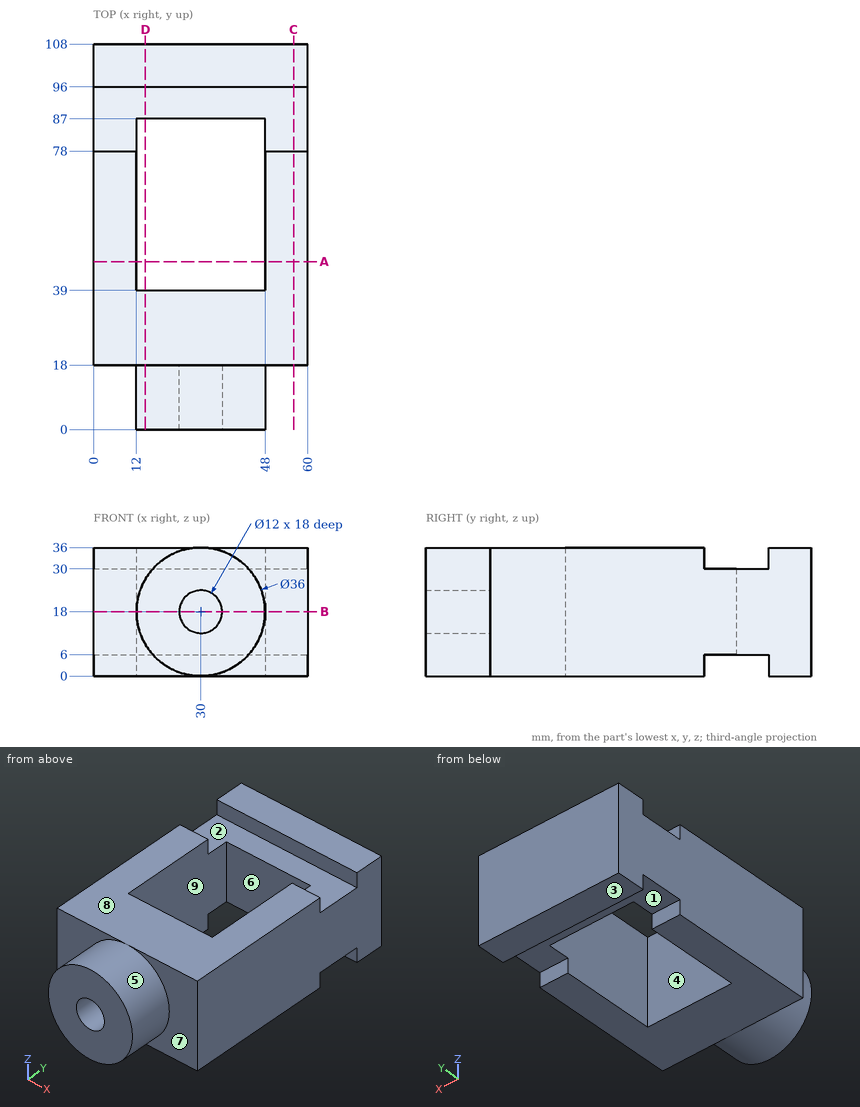
For this review, use the dimensioned drawing (mm, ordinates from the lowest corner) and the shaded views. A direction names the side the tool comes from. Coordinates: 2 decimals unless noted, no trailing zeros. Write each loop counter-clockwise with the first axis right and the second up, starting at its lowest first coordinate (ties: lowest second). Pieces come first, ordered by that corner, then holes. Notation, with made-up numbers: (-36.75, 25) - (16.25, 25) arc R26 cw to (16.25, 62) - close; hole circle Ø4 at (58.5, 24). An arc over 180 degrees is marked (long way). One line per item, written item: value.
1) Add section D-D (x = 14.5). State the section outline as (y, z) points, plus the area to 3 significant figures.
Answer sheet:
outline: (0, 8.85) - (18, 8.85) - (18, 0) - (39, 0) - (39, 36) - (18, 36) - (18, 27.15) - (0, 27.15) - close; (87, 6) - (96, 6) - (96, 0) - (108, 0) - (108, 36) - (96, 36) - (96, 30) - (87, 30) - close
area: 1,730 mm2
2) For the marked faces 1, 2, 3, 4 and 5, list the 3-axis set-ups (+Z, -Z, +X, -X, +Y, -Y) from which the entire face can be reached by the end or side of a thin tool; tool diameter is ignored.
Answer sheet:
face 1: -Z, +X, -X
face 2: +Z, +X, -X
face 3: -Z, +X, -X, +Y, -Y
face 4: +Z, -Z
face 5: -Y
3) Add section C-C (x = 56). State the section outline as (y, z) points, plus the area to 3 significant figures.
Answer sheet:
outline: (18, 0) - (78, 0) - (78, 6) - (96, 6) - (96, 0) - (108, 0) - (108, 36) - (96, 36) - (96, 30) - (78, 30) - (78, 36) - (18, 36) - close
area: 3,020 mm2
4) Add section B-B (z = 18). State the section outline as (x, y) points.
Answer sheet:
outline: (0, 18) - (12, 18) - (12, 0) - (24, 0) - (24, 18) - (36, 18) - (36, 0) - (48, 0) - (48, 18) - (60, 18) - (60, 108) - (0, 108) - close; hole (12, 39) - (48, 39) - (48, 87) - (12, 87) - close
5) To check wall thickness, follow probe 1 along X at (y, z) = (46.5, 21); probe 2 along Z at (x, y) = (30, 6); probe 3 along Y at (x, z) = (18, 8). State the ranges of each line that lie inside material, in increasing order.
Answer sheet:
probe 1: x = 0 to 12, 48 to 60
probe 2: z = 0 to 12, 24 to 36
probe 3: y = 0 to 39, 87 to 108
6) Add section A-A (y = 47). State the section outline as (x, z) points, plus the area to 3 significant figures.
Answer sheet:
outline: (0, 0) - (12, 0) - (12, 36) - (0, 36) - close; (48, 0) - (60, 0) - (60, 36) - (48, 36) - close
area: 864 mm2
7) Insertion check: pin 1 (9 mm diameter, centred on x = 8, z = 15, fed in from -Y); pin 2 (3 mm diameter, centred on x = 41.5, z = 2, fed in from -Y); pin 3 (4 mm diameter, centred on x = 52, y = 88.5, fed in from -Z). Each pin has a flat end and moves straight along its axis. Give the tip position at first contact, or say it passes through.
Answer sheet:
pin 1: stops at y = 0
pin 2: stops at y = 18
pin 3: stops at z = 6
8) Mouldability with a two-part tool opening along Y and no side actions: class the marked faces 6, 7, 8 and 9 as +Y half, -Y half, draft (parallel to the pull), parting line (faces both ways), or undercut.
Answer sheet:
face 6: undercut
face 7: -Y half
face 8: draft
face 9: undercut
